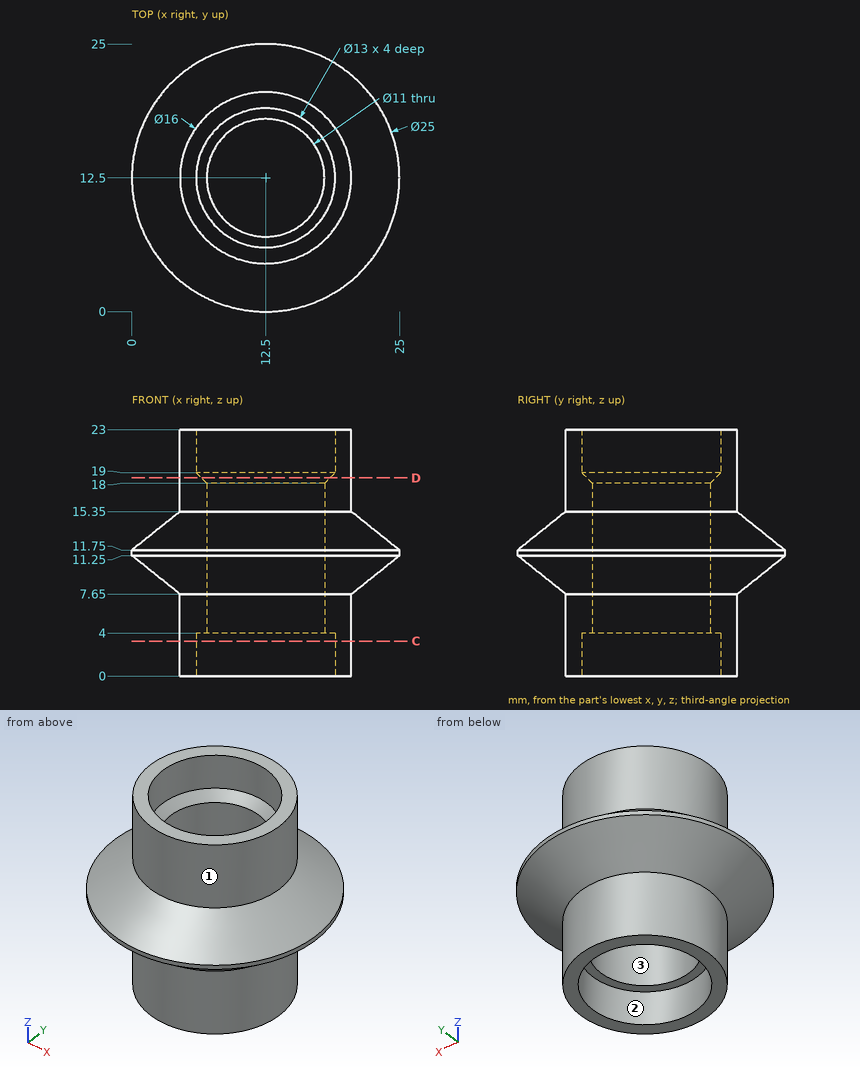
The figure shows three views and two pictorial views of one solid part (mm, origin at its lowest corner). Answer the questions. A direction names the side the tool comes from. Coordinates: 2 decimals unless noted, no trailing zeros. Loops run counter-clockwise (first coordinate to the right, second up) from the corner with the lowest first, then second, coordinate; pieces in that order, holes last.
1) Find section C-C on z = 3.25. Write down the section's boundary in (x, y), then the cut area to 3 significant figures.
2) A tool of negligible diameter and unlimited length cuts with its end or side. For the marked faces 1, 2 and 3, from which of +Z, -Z, +X, -X, +Y, -Y can it reach the whole face along a straight path? Write none if from no direction.
3) Find the intervals of material crossed by L1, parallel to Y at x = 12.5, z = 19.95; L2, parallel to Y at x = 15, z = 11; L3, parallel to X at y = 17.5, z = 20.5 (3 decimals), in increasing order.
4) Flat-ended cylindrical pins translate along their axes: pin 1 Ø3 at (x, y) = (14.5, 11) entering from +Z; pin 2 Ø2 at (y, z) = (12.5, 13.5) entering from +X; pin 3 Ø1.5 at (x, y) = (6.5, 15) entering from -Z; pin 4 Ø11.5 at (x, y) = (12.5, 12.5) entering from -Z. Find the tip coordinate at first contact, or state that the pin passes through.
5) Find section D-D on z = 18.5. Write down the section's boundary in (x, y), then the cut area to 3 significant figures.
Values:
1. outline: circle Ø16 at (12.5, 12.5); hole circle Ø13 at (12.5, 12.5)
1. area: 68.3 mm2
2. face 1: +Z
2. face 2: -Z
2. face 3: +Z, -Z
3. L1: y = 4.5 to 6, 19 to 20.5
3. L2: y = 0.57 to 7.6, 17.4 to 24.43
3. L3: x = 6.255 to 8.347, 16.653 to 18.745
4. pin 1: passes through
4. pin 2: stops at x = 24.06
4. pin 3: stops at z = 0
4. pin 4: stops at z = 4
5. outline: circle Ø16 at (12.5, 12.5); hole circle Ø12 at (12.5, 12.5)
5. area: 88.0 mm2
